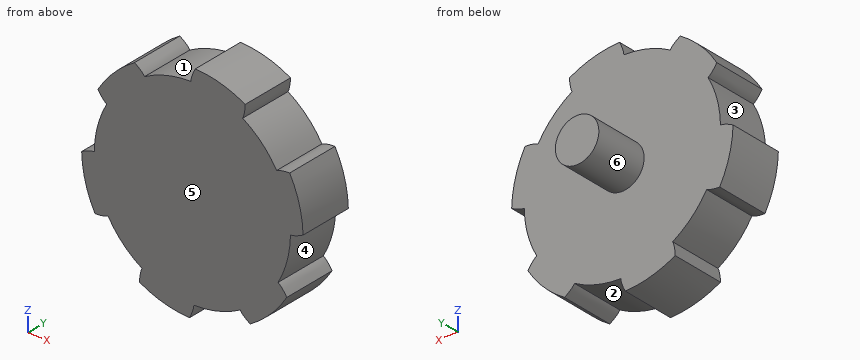
```python
from build123d import *

# Parameters (mm, degrees)
SKETCH_1_R               = 18.042098319
EXTRUDE_1_DEPTH          = 10
EXTRUDE_2_DEPTH          = 10
PATTERN_CIRCULAR_1_COUNT = 6
SKETCH_5_R               = 4
EXTRUDE_3_DEPTH          = 10


with BuildPart() as part:
    # ｽｹｯﾁ1 → ﾎﾞｽ - 押し出し1 (new body)
    with BuildSketch(Plane(origin=(0, 0, 0), x_dir=(1, 0, 0), z_dir=(0, 1, 0))):
        with Locations(Location((0, 0, 0), (0, 0, 270))):
            Circle(SKETCH_1_R)
    extrude(amount=EXTRUDE_1_DEPTH)

    # ｽｹｯﾁ4 → ﾎﾞｽ - 押し出し2 (add)
    with BuildSketch(Plane(origin=(0, 0, 0), x_dir=(1, 0, 0), z_dir=(0, 1, 0))):
        with BuildLine():
            ThreePointArc((0.268896403, 18.040094414), (-4.669638659, 17.427328727), (-9.252918324, 15.488731848))
            add(Edge.make_bspline(
                [(-9.714533079, 17.890556389), (-9.709818433, 17.598094858), (-9.683773216, 17.175123253), (-9.606482839, 16.645312354), (-9.53966415, 16.315628537), (-9.468789573, 16.043783597), (-9.40010103, 15.828997964), (-9.331330572, 15.648985933), (-9.28257301, 15.54191839), (-9.252918324, 15.488731848)],
                knots=[0, 0, 0, 0, 0.356146416, 0.515080655, 0.651524593, 0.765478231, 0.856941573, 0.925914628, 1, 1, 1, 1], degree=3))
            ThreePointArc((-9.714533079, 17.890556389), (-5.269012673, 19.664223003), (-0.532245762, 20.35094286))
            add(Edge.make_bspline(
                [(-0.532245762, 20.35094286), (-0.390098, 20.095306422), (-0.201168016, 19.715979658), (-0.003197997, 19.218504772), (0.103777229, 18.899580866), (0.178320514, 18.628718954), (0.226227308, 18.408364869), (0.25667636, 18.218084648), (0.267984844, 18.100982654), (0.268896403, 18.040094414)],
                knots=[0, 0, 0, 0, 0.356146416, 0.515080655, 0.651524593, 0.765478231, 0.856941573, 0.925914628, 1, 1, 1, 1], degree=3))
        make_face()
    extrude_2 = extrude(amount=EXTRUDE_2_DEPTH)

    # 円形ﾊﾟﾀｰﾝ1: ﾎﾞｽ - 押し出し2 ×6 about axis
    pattern_circular_1_axis = Axis((0, 10, 0), (0, 1, 0))
    for i in range(1, PATTERN_CIRCULAR_1_COUNT):
        add(extrude_2.rotate(pattern_circular_1_axis, i * 360 / PATTERN_CIRCULAR_1_COUNT))

    # ｽｹｯﾁ5 → ﾎﾞｽ - 押し出し3 (add)
    with BuildSketch(Plane(origin=(0, 10, 0), x_dir=(1, 0, 0), z_dir=(0, 1, 0))):
        with Locations(Location((0, 0, 0), (0, 0, 270))):
            Circle(SKETCH_5_R)
    extrude(amount=EXTRUDE_3_DEPTH)


solid = part.part
```
Read the model definition and answer for the solid it produces. Units are mm, in the model's axes. Face numbers are marked on the shaded views. A direction names the side the tool comes from. Give positions to 0.01 mm unless a question says otherwise; leave off trailing zeros. Order: outer loops, then holes, each group sorted by start corner. A loop starts at its lowest first (then second) coordinate and runs counter-clockwise, first axis right, second up. Notation, with made-up numbers: (40, 68) -> (62, 68) arc R29 cw to (62, 102) -> close; hole circle Ø4 at (31, 51.5). An arc over 180 degrees is marked (long way). Write item = value, one per line.
1. For the marked faces 5 and 6, determine the directions among +Z, -Z, +X, -X, +Y, -Y from which every point of the face is accessible in a straight line to the end or side of a thin tool.
Numbers:
face_5 = +Z, -Z, +X, -X, -Y
face_6 = +Y
2. A cutting plane is placed at D-D, the plane x = 15. Write down the section's boundary in (y, z), and give its area (3 significant figures).
Numbers:
outline = (0, -13.76) -> (10, -13.76) -> (10, 10.03) -> (0, 10.03) -> close
area = 238 mm²
3. A cutting plane is placed at A-A, the plane y = 12. Write down the section's boundary in (x, z), and give its area (3 significant figures).
Numbers:
outline = circle Ø8 at (0, 0)
area = 50.3 mm²
4. Straight lines are drawn through the part: line 1 along Y through (x, z) = (-14.5, 3); line 2 along X through (y, z) = (5.75, 6); line 3 along Z through (x, y) = (11.5, 3.75). For each, find the intervals that lie inside material, in ascending order.
Numbers:
line_1 = 0 to 10
line_2 = -17.02 to 19.45
line_3 = -16.8 to 13.9
5. A cutting plane is placed at C-C, the plane z = 7.5. Write down the section's boundary in (x, y), and give its area (3 significant figures).
Numbers:
outline = (-16.41, 0) -> (18.93, 0) -> (18.93, 10) -> (-16.41, 10) -> close
area = 353 mm²
6. A cutting plane is placed at B-B, the plane x = -3.5. Write down the section's boundary in (y, z), and give its area (3 significant figures).
Numbers:
outline = (0, -20.05) -> (10, -20.05) -> (10, -1.94) -> (20, -1.94) -> (20, 1.94) -> (10, 1.94) -> (10, 17.7) -> (0, 17.7) -> close
area = 416 mm²
7. Given pin 1 (1 mm diameter, centred on x = 3.5, z = 11, fed in from +Y); pin 2 (4 mm diameter, centred on y = 3.5, z = 14, fed in from -X); pin 3 (3 mm diameter, centred on x = 12.5, z = 10.5, fed in from -Y); pin 4 (4 mm diameter, centred on x = -9, y = 8, fed in from -Z), each flat-ended and moving along its own axis, determine where each tip first touches the part or whether it passes through.
Numbers:
pin_1 = 10
pin_2 = -16.45
pin_3 = 0
pin_4 = -19.12
8. The mould has two halves that part along X. Classify the marked faces 1, 2, 3 and 4: +X half, -X half, draft (parallel to the pull), parting line (faces both ways), or undercut.
Numbers:
face_1 = undercut
face_2 = undercut
face_3 = -X half
face_4 = +X half
